```python
from build123d import *

# Parameters (mm, degrees)
SKETCH2_W           = 6.2
SKETCH2_H           = 4
BOSS_EXTRUDE1_DEPTH = 6.2
CUT_EXTRUDE1_DEPTH  = 1


with BuildPart() as part:
    # Sketch2 → Boss-Extrude1 (new body)
    with BuildSketch(Plane(origin=(0, 0, 0), x_dir=(1, 0, 0), z_dir=(0, 1, 0))):
        Polygon((-0.1, 7), (6.2, 7), (31.2, 7), (31.2, -3), (6.2, -3), (-0.1, -3), (-11.95, -3), (-11.95, 7), align=None)
        with Locations((3.1, 2)):
            Rectangle(SKETCH2_W, SKETCH2_H, mode=Mode.SUBTRACT)
    extrude(amount=BOSS_EXTRUDE1_DEPTH)

    # Sketch3 → Cut-Extrude1 (cut)
    with BuildSketch(Plane(origin=(0, 6.2, 0), x_dir=(1, 0, 0), z_dir=(0, 1, 0))):
        with BuildLine():
            Line((19.276089489, 0.490389836), (19.048395179, 0.648758226))
            Line((19.048395179, 0.648758226), (19.931187647, 1.939237994))
            add(Edge.make_bspline(
                [(19.931187647, 1.939237994), (19.874862479, 1.93235), (19.763955085, 1.918787158), (19.652252142, 1.91629555), (19.597278392, 1.915069324)],
                knots=[0, 0, 0, 0, 0.000170115, 0.000334967, 0.000334967, 0.000334967, 0.000334967], degree=3))
            add(Edge.make_bspline(
                [(19.597278392, 1.915069324), (19.563948105, 1.915923014), (19.498523668, 1.917598735), (19.402337812, 1.930880947), (19.309913054, 1.951337134), (19.221494424, 1.981861362), (19.136749587, 2.019796451), (19.055863547, 2.066838171), (18.978945189, 2.122179593), (18.90682061, 2.185528092), (18.841223533, 2.25508604), (18.782782398, 2.328705801), (18.734212943, 2.407242575), (18.693866326, 2.489094274), (18.663267986, 2.575437356), (18.640986256, 2.665289312), (18.62726812, 2.759279873), (18.625636083, 2.823256242), (18.624807438, 2.855739396)],
                knots=[0, 0, 0, 0, 9.9954e-05, 0.000196201, 0.000290782, 0.000383503, 0.000476303, 0.000568919, 0.000663705, 0.000760153, 0.000856434, 0.000950205, 0.001041624, 0.001132931, 0.001223461, 0.001315861, 0.001410305, 0.001507717, 0.001507717, 0.001507717, 0.001507717], degree=3))
            add(Edge.make_bspline(
                [(18.624807438, 2.855739396), (18.626380818, 2.900160959), (18.629469044, 2.987351477), (18.654323414, 3.114744968), (18.695199578, 3.235201332), (18.752193892, 3.348403865), (18.823980389, 3.45272415), (18.910257467, 3.54671196), (19.010500349, 3.629030506), (19.122425466, 3.699791348), (19.243395707, 3.756700952), (19.370095132, 3.798646603), (19.501552941, 3.823319753), (19.590605042, 3.826572641), (19.635439449, 3.828210349)],
                knots=[0, 0, 0, 0, 0.000133185, 0.000261414, 0.000387724, 0.00051373, 0.000640399, 0.00076644, 0.000895188, 0.001028407, 0.001162697, 0.001295241, 0.001427846, 0.0015623, 0.0015623, 0.0015623, 0.0015623], degree=3))
            add(Edge.make_bspline(
                [(19.635439449, 3.828210349), (19.679425373, 3.82655013), (19.766337412, 3.823269693), (19.894143868, 3.79924495), (20.016554647, 3.758753111), (20.132891171, 3.702796399), (20.240604781, 3.63265529), (20.337465695, 3.549076115), (20.421263506, 3.452006815), (20.491860883, 3.343795114), (20.548530134, 3.227529352), (20.589417134, 3.106168222), (20.614586392, 2.980584525), (20.61775806, 2.895499538), (20.61935872, 2.852559308)],
                knots=[0, 0, 0, 0, 0.000131915, 0.000260652, 0.000388569, 0.000517718, 0.000646848, 0.000773094, 0.000900237, 0.001030248, 0.001159674, 0.001287189, 0.001413545, 0.001542287, 0.001542287, 0.001542287, 0.001542287], degree=3))
            add(Edge.make_bspline(
                [(20.61935872, 2.852559308), (20.618289735, 2.819227462), (20.616121566, 2.75162215), (20.600939344, 2.648906053), (20.575158176, 2.544175295), (20.545901278, 2.455527847), (20.517659955, 2.382313754), (20.491079642, 2.324481963), (20.461586475, 2.263611531), (20.427188737, 2.200340732), (20.390211511, 2.133863004), (20.348429167, 2.064845112), (20.302794827, 1.993194439), (20.270292153, 1.944891724), (20.253648584, 1.920157465)],
                knots=[0, 0, 0, 0, 9.9984e-05, 0.000202793, 0.000310776, 0.000423207, 0.000482616, 0.000546097, 0.000614079, 0.0006855, 0.000762103, 0.000842274, 0.000927493, 0.001016928, 0.001016928, 0.001016928, 0.001016928], degree=3))
            Line((20.253648584, 1.920157465), (19.276089489, 0.490389836))
        make_face()
        with BuildLine():
            add(Edge.make_bspline(
                [(19.650067855, 2.240710349), (19.675317282, 2.241400126), (19.724469333, 2.242742887), (19.796475883, 2.250915556), (19.864442839, 2.265406244), (19.928551758, 2.286197697), (19.989445447, 2.311286246), (20.046156688, 2.343228548), (20.098732942, 2.381343638), (20.147526275, 2.424169867), (20.190855047, 2.471750039), (20.229447653, 2.521549557), (20.262250454, 2.573787025), (20.288161426, 2.629116627), (20.309465291, 2.686191523), (20.324177345, 2.745930831), (20.332327419, 2.808023309), (20.333716776, 2.850204234), (20.334422823, 2.871639836)],
                knots=[0, 0, 0, 0, 7.5753e-05, 0.000147465, 0.000217073, 0.000283852, 0.000349411, 0.000414338, 0.000478589, 0.000543925, 0.000608743, 0.000671332, 0.000732749, 0.000793345, 0.000854313, 0.000915245, 0.00097749, 0.001041807, 0.001041807, 0.001041807, 0.001041807], degree=3))
            add(Edge.make_bspline(
                [(20.334422823, 2.871639836), (20.333815337, 2.89308439), (20.332618212, 2.935343513), (20.323014019, 2.99752792), (20.306118281, 3.057121092), (20.283448341, 3.114449282), (20.253584983, 3.169041477), (20.217749678, 3.221583075), (20.175175241, 3.271740933), (20.126187199, 3.318335404), (20.07336014, 3.361286713), (20.017062401, 3.399192653), (19.957758012, 3.430961881), (19.895808782, 3.457177375), (19.831085637, 3.477635058), (19.763626877, 3.492346524), (19.693091616, 3.500485187), (19.645211449, 3.501865763), (19.620811044, 3.502569324)],
                knots=[0, 0, 0, 0, 6.4316e-05, 0.000126743, 0.000188161, 0.000249812, 0.000311283, 0.000374438, 0.00044032, 0.000508243, 0.00057698, 0.000644365, 0.000711521, 0.0007785, 0.000845884, 0.000914871, 0.00098532, 0.001058531, 0.001058531, 0.001058531, 0.001058531], degree=3))
            add(Edge.make_bspline(
                [(19.620811044, 3.502569324), (19.596622848, 3.501864626), (19.549165806, 3.500482016), (19.479257604, 3.492361994), (19.412254973, 3.477536119), (19.347719361, 3.457186851), (19.285771971, 3.430959926), (19.22647038, 3.399190988), (19.170159472, 3.361295438), (19.117383061, 3.318301609), (19.068308518, 3.271957816), (19.026466073, 3.221363348), (18.990548757, 3.169068808), (18.960726433, 3.114442018), (18.938045578, 3.057123031), (18.921152762, 2.997527395), (18.911547784, 2.93534365), (18.910350767, 2.893084436), (18.909743336, 2.871639836)],
                knots=[0, 0, 0, 0, 7.2576e-05, 0.000142393, 0.000210758, 0.000278143, 0.000345121, 0.000412278, 0.000479663, 0.0005484, 0.000616323, 0.000681795, 0.00074495, 0.000806421, 0.000868072, 0.00092949, 0.000991917, 0.001056233, 0.001056233, 0.001056233, 0.001056233], degree=3))
            add(Edge.make_bspline(
                [(18.909743336, 2.871639836), (18.910292997, 2.850187542), (18.91137703, 2.807879691), (18.921834382, 2.745716463), (18.939322536, 2.686127887), (18.962744412, 2.62853456), (18.993588712, 2.573496517), (19.031438202, 2.521274696), (19.075802519, 2.471277109), (19.126088611, 2.424280567), (19.1811233, 2.38114395), (19.239903206, 2.343469961), (19.301416415, 2.311654244), (19.365879466, 2.286125988), (19.432814634, 2.265613979), (19.502823503, 2.250942263), (19.575674547, 2.242821278), (19.625032174, 2.241420743), (19.650067855, 2.240710349)],
                knots=[0, 0, 0, 0, 6.4316e-05, 0.000126844, 0.000188436, 0.000250326, 0.000312966, 0.000377217, 0.000443451, 0.000513196, 0.000583426, 0.000652939, 0.000722346, 0.000790847, 0.000860662, 0.000932137, 0.001005113, 0.00108023, 0.00108023, 0.00108023, 0.00108023], degree=3))
        make_face(mode=Mode.SUBTRACT)
        Polygon((21.229935643, 3.746800093), (23.183781797, 3.746800093), (21.514871541, 0.490389836), (21.268732719, 0.625861591), (22.701680435, 3.421159067), (21.229935643, 3.421159067), align=None)
    extrude(amount=-CUT_EXTRUDE1_DEPTH, mode=Mode.SUBTRACT)


solid = part.part
```
Check sheet for the modelled part. Datum: model origin and axes. Units: mm. A direction names the side the tool comes from. Give positions to 0.01 mm unless a question says otherwise; leave off trailing zeros. Order: outer loops, then holes, each group sorted by start corner. A loop starts at its lowest first (then second) coordinate and runs counter-clockwise, first axis right, second up. Notation, with made-up numbers: M 41,65.5 L 50,65.5 A20 ccw 50,90.5 Z; hole C -2,2.25 d1. An arc over 180 degrees is marked long. Answer in a Markdown table with one row per item. Add a question column.
Q1. Sectioned sample at C-C, the plane z = -1.5. Record the boundary of the cut face in (x, y), and give its area (3 significant figures).
Q2. Sectioned sample at B-B, the plane y = 1.5. Record the boundary of the cut face in (x, z).
Q3. Access from +Z, -Z, +X, -X, +Y, -Y to the whole of each face (thin tool, end or side, straight path). Record for faces 1 (the flat face through (10, 0, -2)), 2 (the flat face through (22.36, 5.71, -2.14)), 3 (the flat face through (6.2, 3, -2)).
Q4. Sectioned sample at A-A, the plane x = 2. Record the boundary of the cut face in (y, z).
Q5. Thickness scan on L1, parallel to X at y = 1, z = -3.5; L2, parallel to Z at x = 1.5, y = 4.75; L3, parallel to X at y = 5.25, z = -1.25. Record the ranges inside material, lowest first.
Q6. Release check for a two-part mould opening along X. For faces 4 (the flat face through (22, 6, -3.421)), 5 (the flat face through (31.2, 3, -2)), 6 (the flat face through (10, 3, -7)), 7 (the flat face through (21.975, 5.707, -2.004)) record: released by +X, released by -X, zero draft, split by the parting line, or undercut.
Verdict:
| question | item | result |
|---|---|---|
| 1 | outline | M -11.95,0 L 0,0 L 0,6.2 L -11.95,6.2 Z; M 6.2,0 L 31.2,0 L 31.2,6.2 L 22.03,6.2 L 22.03,5.2 L 21.72,5.2 L 21.72,6.2 L 19.97,6.2 L 19.97,5.2 L 19.63,5.2 L 19.63,6.2 L 6.2,6.2 Z |
| 1 | area | 228 mm² |
| 2 | outline | M -11.95,-7 L 31.2,-7 L 31.2,3 L -11.95,3 Z; hole M 0,-4 L 6.2,-4 L 6.2,0 L 0,0 Z |
| 3 | face 1 | +Z, -Z, +X, -X, -Y |
| 3 | face 2 | +Y |
| 3 | face 3 | +Y, -Y |
| 4 | outline | M 0,-7 L 6.2,-7 L 6.2,-4 L 0,-4 Z; M 0,0 L 6.2,0 L 6.2,3 L 0,3 Z |
| 5 | L1 | -11.95 to 0, 6.2 to 31.2 |
| 5 | L2 | -7 to -4, 0 to 3 |
| 5 | L3 | -11.95 to 0, 6.2 to 19.46, 19.8 to 21.59, 21.9 to 31.2 |
| 6 | face 4 | undercut |
| 6 | face 5 | released by +X |
| 6 | face 6 | zero draft |
| 6 | face 7 | undercut |
